Here's the drawing with two shaded views (mm, measured from the low corner). I have some questions. A direction names the side the tool comes from. Round coordinates to 2 decimals unless told otherwise and drop trailing zeros. Loops run counter-clockwise (first coordinate to the right, second up) from the corner with the lowest first, then second, coordinate; pieces in that order, holes last. Notation, with made-up numbers: (56.5, 15.5) - (71.5, 15.5) arc R28 cw to (71.5, 53.5) - close; hole circle Ø6 at (68.5, 82.5). An arc over 180 degrees is marked (long way). Use one line per item in the form item = value.
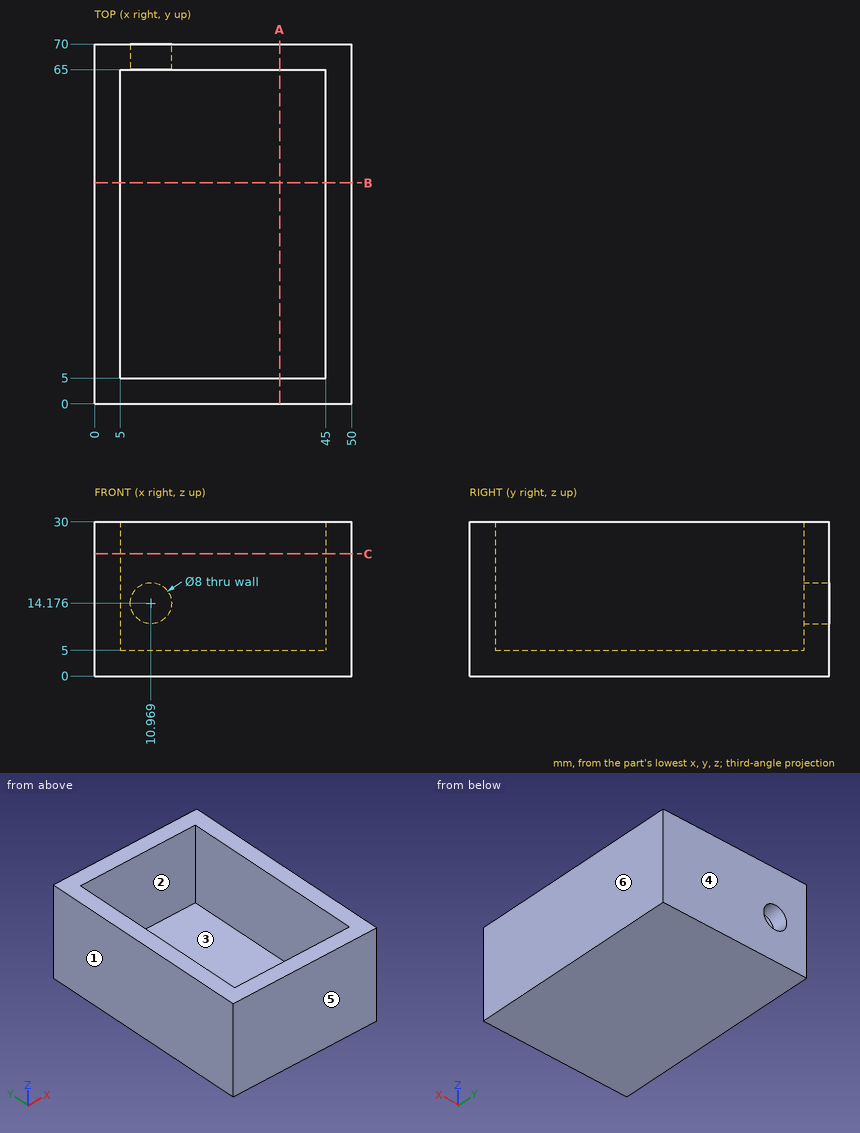
1. If we section it at C-C, the plane z = 23.75: Write out the boundary of the cut face in (x, y), plus the area to 3 significant figures.
Solution:
outline = (0, 0) - (50, 0) - (50, 70) - (0, 70) - close; hole (5, 5) - (45, 5) - (45, 65) - (5, 65) - close
area = 1,100 mm^2
2. On a 3-axis mill with a long thin cutter (end or side, diameter ignored), from which of +Z, -Z, +X, -X, +Y, -Y can I reach the whole of each face in a straight line? I mean the marked faces 1 and 2. Say none if no direction works.
Solution:
face_1 = +Z, -Z, -X, +Y, -Y
face_2 = +Z
3. For P1, Ø12, axis at x = 25.5, y = 54.5, coming from the -Z side; P2, Ø7, axis at x = 10.97, z = 14.18, coming from the +Y side; P3, Ø1.5, axis at x = 13, y = 18, coming from the +Z side, each with a flat end and sliding along its axis, tell me the tip position at first contact or that it passes through.
Solution:
P1 = 0
P2 = 5
P3 = 5
4. If we section it at B-B, the plane y = 43: Write out the boundary of the cut face in (x, z), plus the area to 3 significant figures.
Solution:
outline = (0, 0) - (50, 0) - (50, 30) - (45, 30) - (45, 5) - (5, 5) - (5, 30) - (0, 30) - close
area = 500 mm^2
5. Please list where these lines run through material, in increasing order: line 1 along X through (y, z) = (47, 10.5); line 2 along Y through (x, z) = (26.5, 24.5); line 3 along Z through (x, y) = (17, 34).
Solution:
line_1 = 0 to 5, 45 to 50
line_2 = 0 to 5, 65 to 70
line_3 = 0 to 5
6. We'd pull the mould along Y, two halves only. Please class the marked faces 3, 4, 5 and 6: +Y half, -Y half, draft (parallel to the pull), parting line (faces both ways), or undercut.
Solution:
face_3 = undercut
face_4 = +Y half
face_5 = -Y half
face_6 = draft
7. If we section it at A-A, the plane x = 36: Write out the boundary of the cut face in (y, z), plus the area to 3 significant figures.
Solution:
outline = (0, 0) - (70, 0) - (70, 30) - (65, 30) - (65, 5) - (5, 5) - (5, 30) - (0, 30) - close
area = 600 mm^2
